Source: CAD feature listing. Evaluate the final solid. Frame: model axes, mm. A direction names the side the tool comes from. Give positions to 0.01 mm unless a question says otherwise; leave off trailing zeros. Order: outer loops, then holes, each group sorted by start corner. A loop starts at its lowest first (then second) coordinate and runs counter-clockwise, first axis right, second up. Notation, with made-up numbers: (-38, 8.25) -> (10, 8.25) arc R19 cw to (10, 23.25) -> close; hole circle Ø7 at (21.25, -23). An arc over 180 degrees is marked (long way). Use one line per item in the form item = value. Start each with the question number.
from build123d import *

# Parameters (mm, degrees)
SKETCH1_R           = 1.5
SKETCH1_R_2         = 1.500000075
SKETCH1_R_3         = 1.499999926
BOSS_EXTRUDE1_DEPTH = 2


with BuildPart() as part:
    # Sketch1 → Boss-Extrude1 (new body)
    with BuildSketch(Plane(origin=(0, 0, 0), x_dir=(1, 0, 0), z_dir=(0, 1, 0))):
        with BuildLine():
            Line((16.641623692, -1.328817394), (16.641623692, -16.412584868))
            ThreePointArc((16.641623692, -16.412584868), (16.946106169, -17.943318476), (17.813197688, -19.241011527))
            Line((17.813197688, -19.241011527), (20.073605121, -21.501420823))
            ThreePointArc((20.073605121, -21.501420823), (20.073603258, -27.865380806), (13.709643275, -27.865378943))
            Line((13.709643275, -27.865378943), (10.626761594, -24.782500056))
            ThreePointArc((10.626761594, -24.782500056), (9.329068113, -23.915408358), (7.798334003, -23.610926059))
            Line((7.798334003, -23.610926059), (-9.015085756, -23.610926059))
            ThreePointArc((-9.015085756, -23.610926059), (-10.545819865, -23.915408358), (-11.843513346, -24.782500056))
            Line((-11.843513346, -24.782500056), (-14.926395028, -27.865378943))
            ThreePointArc((-14.926395028, -27.865378943), (-21.290355011, -27.865380806), (-21.290356874, -21.501420823))
            Line((-21.290356874, -21.501420823), (-19.029949441, -19.241011527))
            ThreePointArc((-19.029949441, -19.241011527), (-18.162857921, -17.943318476), (-17.858375444, -16.412584868))
            Line((-17.858375444, -16.412584868), (-17.858375444, -1.328817394))
            ThreePointArc((-17.858375444, -1.328817394), (-17.9789903, -0.644777024), (-18.326286807, -0.043242064))
            Line((-18.326286807, -0.043242064), (-23.644334286, 6.294557068))
            ThreePointArc((-23.644334286, 6.294557068), (-23.650520639, 6.302037606), (-23.656743228, 6.309488031))
            Line((-23.656743228, 6.309488031), (-24.213413357, 6.972902629))
            ThreePointArc((-24.213413357, 6.972902629), (-24.650941114, 7.911183978), (-24.560709133, 8.942523214))
            Line((-24.560709133, 8.942523214), (-22.191124617, 15.452907595))
            ThreePointArc((-22.191124617, 15.452907595), (-21.597313109, 16.300951983), (-20.659035652, 16.738475475))
            Line((-20.659035652, 16.738475475), (-19.806167691, 16.888857993))
            ThreePointArc((-19.806167691, 16.888857993), (-18.867887285, 17.3263878), (-18.274078726, 18.174440774))
            Line((-18.274078726, 18.174440774), (-15.59413655, 25.537521753))
            ThreePointArc((-15.59413655, 25.537521753), (-14.129671055, 27.446048523), (-11.835365205, 28.169439348))
            Line((-11.835365205, 28.169439348), (10.618613453, 28.169439348))
            ThreePointArc((10.618613453, 28.169439348), (12.912919302, 27.446048523), (14.377384798, 25.537521753))
            Line((14.377384798, 25.537521753), (17.057326973, 18.174440774))
            ThreePointArc((17.057326973, 18.174440774), (17.651135533, 17.3263878), (18.589415939, 16.888857993))
            Line((18.589415939, 16.888857993), (19.4422839, 16.738475475))
            ThreePointArc((19.4422839, 16.738475475), (20.380561357, 16.300951983), (20.974372865, 15.452907595))
            Line((20.974372865, 15.452907595), (23.34395738, 8.942523214))
            ThreePointArc((23.34395738, 8.942523214), (23.434189362, 7.911183978), (22.996661604, 6.972902629))
            Line((22.996661604, 6.972902629), (22.439991475, 6.309488031))
            ThreePointArc((22.439991475, 6.309488031), (22.433768887, 6.302037606), (22.427582533, 6.294557068))
            Line((22.427582533, 6.294557068), (17.109535054, -0.043242064))
            ThreePointArc((17.109535054, -0.043242064), (16.762238548, -0.644777024), (16.641623692, -1.328817394))
        make_face()
        with Locations((-18.108375876, 10.316600984)):
            Circle(SKETCH1_R, mode=Mode.SUBTRACT)
        with Locations((-18.108375951, -24.683399883)):
            Circle(SKETCH1_R_2, mode=Mode.SUBTRACT)
        with Locations((16.891624198, -24.683399883)):
            Circle(SKETCH1_R_3, mode=Mode.SUBTRACT)
        with Locations((16.891624124, 10.316600984)):
            Circle(SKETCH1_R, mode=Mode.SUBTRACT)
        with BuildLine():
            Line((-14.858375884, -17.61092135), (-14.858375884, 6.889076146))
            ThreePointArc((-14.858375884, 6.889076146), (-14.272588129, 8.303287628), (-12.858375556, 8.889072749))
            Line((-12.858375556, 8.889072749), (11.641623803, 8.889072749))
            ThreePointArc((11.641623803, 8.889072749), (13.055836377, 8.303287628), (13.641624131, 6.889076146))
            Line((13.641624131, 6.889076146), (13.641624131, -17.61092135))
            ThreePointArc((13.641624131, -17.61092135), (13.055839011, -19.025137649), (11.641623803, -19.610925403))
            Line((11.641623803, -19.610925403), (-12.858375556, -19.610925403))
            ThreePointArc((-12.858375556, -19.610925403), (-14.272590763, -19.025137649), (-14.858375884, -17.61092135))
        make_face(mode=Mode.SUBTRACT)
    extrude(amount=BOSS_EXTRUDE1_DEPTH)


solid = part.part
1) Cut plane C-C, the plane z = -11. Return the cut outline in (x, y), plus the area to 3 significant figures.
2) Cut plane B-B, the plane x = 0.5. Return the cut outline in (y, z), plus the area to 3 significant figures.
3) Cut plane A-A, the plane z = 11. Return the cut outline in (x, y), plus the area to 3 significant figures.
4) Draft query along Z for faces 6 (the face through (-23.393, 0.986, -12.152)), 7 (the face through (-14.858, 1, 6)), 8 (the face through (9.349, 0.986, 23.924)). Return one class per face: +Z half, -Z half, draft (parallel to the pull), parting line (faces both ways), or undercut.
5) Cut plane D-D, the plane y = 0.65. Count the separate pieces of the cut face and the enclosed holes in it, plus the area to 3 significant figures.
6) Material intervals for probe 1 along Z at (x, y) = (-2, 0.3); probe 2 along X at (y, z) = (0.45, 15); probe 3 along Z at (x, y) = (-19, 0.3), sorted ascending.
7) Reachability of faces 1 (the face through (0, 1, 23.611)), 2 (the face through (-1, 1, -28.169)), 3 (the face through (19.806, 0.986, -3.17)), 4 (the face through (-18.17, 0.99, 17.96)), 5 (the face through (13.04, 0.99, -8.32)) from +Z, -Z, +X, -X, +Y, -Y: full face, straight path, thin tool, end or side. Return the list, or none.
Output values:
q1.outline = (-23.81, 0) -> (-19.44, 0) -> (-19.44, 2) -> (-23.81, 2) -> close; (-16.77, 0) -> (15.56, 0) -> (15.56, 2) -> (-16.77, 2) -> close; (18.23, 0) -> (22.6, 0) -> (22.6, 2) -> (18.23, 2) -> close
q1.area = 82.1 mm^2
q2.outline = (0, -28.17) -> (2, -28.17) -> (2, -8.89) -> (0, -8.89) -> close; (0, 19.61) -> (2, 19.61) -> (2, 23.61) -> (0, 23.61) -> close
q2.area = 46.6 mm^2
q3.outline = (-17.86, 0) -> (-14.86, 0) -> (-14.86, 2) -> (-17.86, 2) -> close; (13.64, 0) -> (16.64, 0) -> (16.64, 2) -> (13.64, 2) -> close
q3.area = 12.0 mm^2
q4.face_6 = -Z half
q4.face_7 = undercut
q4.face_8 = +Z half
q5.separate_pieces = 1
q5.enclosed_holes = 5
q5.area = 1,200 mm^2
q6.probe_1 = -28.17 to -8.89, 19.61 to 23.61
q6.probe_2 = -17.86 to -14.86, 13.64 to 16.64
q6.probe_3 = -17.22 to -11.52, -9.11 to -0.76, 19.21 to 23.48, 25.89 to 29.09
q7.face_1 = +Z, +Y, -Y
q7.face_2 = -Z, +X, -X, +Y, -Y
q7.face_3 = +X, +Y, -Y
q7.face_4 = -X, +Y, -Y
q7.face_5 = +Y, -Y
